```python
from build123d import *

# Parameters (mm, degrees)
SKETCH2_W           = 304.8
SKETCH2_H           = 304.8
BOSS_EXTRUDE1_DEPTH = 5.588
SKETCH4_W           = 1.27
SKETCH4_H           = 12.7
SKETCH4_W_2         = 12.7
SKETCH4_H_2         = 1.27
CUT_EXTRUDE1_DEPTH  = 432.088512656
SKETCH5_W           = 228.854
SKETCH5_H           = 12.954
CUT_EXTRUDE2_DEPTH  = 0.254
SKETCH6_R           = 16.002
SKETCH6_R_2         = 1.7
SKETCH6_R_3         = 1.96
CUT_EXTRUDE3_DEPTH  = 432.088512656
CUT_EXTRUDE4_DEPTH  = 432.088512656
SKETCH8_R           = 1.016
CUT_EXTRUDE5_DEPTH  = 432.088512656
SKETCH9_R           = 1.016
CUT_EXTRUDE6_DEPTH  = 432.088512656
BOSS_EXTRUDE3_REACH = 433.089
SKETCH10_W          = 236.011664121
SKETCH10_H          = 22.945578457


with BuildPart() as part:
    # Sketch2 → Boss-Extrude1 (new body)
    with BuildSketch(Plane(origin=(0, 0, 0), x_dir=(1, 0, 0), z_dir=(0, 1, 0))):
        with Locations((152.4, 152.4)):
            Rectangle(SKETCH2_W, SKETCH2_H)
    extrude(amount=BOSS_EXTRUDE1_DEPTH)

    # Sketch4 → Cut-Extrude1 (cut, through all)
    with BuildSketch(Plane(origin=(0, 5.588, 0), x_dir=(1, 0, 0), z_dir=(0, 1, 0))):
        with Locations((3.175, 8.89)):
            Rectangle(SKETCH4_W, SKETCH4_H)
        with Locations((295.91, 3.175)):
            Rectangle(SKETCH4_W_2, SKETCH4_H_2)
        with Locations((295.91, 6.985)):
            Rectangle(SKETCH4_W_2, SKETCH4_H_2)
    extrude(amount=-CUT_EXTRUDE1_DEPTH, mode=Mode.SUBTRACT)

    # Sketch5 → Cut-Extrude2 (cut)
    with BuildSketch(Plane(origin=(0, 5.588, 0), x_dir=(1, 0, 0), z_dir=(0, 1, 0))):
        with Locations((148.97354, 274.58924)):
            Rectangle(SKETCH5_W, SKETCH5_H)
    extrude(amount=-CUT_EXTRUDE2_DEPTH, mode=Mode.SUBTRACT)

    # Sketch6 → Cut-Extrude3 (cut, through all)
    with BuildSketch(Plane(origin=(0, 5.588, 0), x_dir=(1, 0, 0), z_dir=(0, 1, 0))):
        with Locations(Location((152.4799846, 126.1262654, 0), (0, 0, 270))):
            Circle(SKETCH6_R)
        with Locations(Location((31.75, 300.959132824, 0), (0, 0, 270))):
            Circle(SKETCH6_R_2)
        with Locations(Location((17.93875, 287.147882824, 0), (0, 0, 270))):
            Circle(SKETCH6_R_2)
        with Locations(Location((273.05, 300.959132824, 0), (0, 0, 270))):
            Circle(SKETCH6_R_2)
        with Locations(Location((286.86125, 287.147882824, 0), (0, 0, 270))):
            Circle(SKETCH6_R_2)
        with Locations(Location((286.86125, 222.906202824, 0), (0, 0, 270))):
            Circle(SKETCH6_R_2)
        with Locations(Location((273.05, 209.094952824, 0), (0, 0, 270))):
            Circle(SKETCH6_R_2)
        with Locations(Location((31.75, 209.094952824, 0), (0, 0, 270))):
            Circle(SKETCH6_R_2)
        with Locations(Location((17.93875, 222.906202824, 0), (0, 0, 270))):
            Circle(SKETCH6_R_2)
        with Locations(Location((38.1787654, 103.9330154, 0), (0, 0, 270))):
            Circle(SKETCH6_R_2)
        with Locations(Location((53.1330154, 88.9787654, 0), (0, 0, 270))):
            Circle(SKETCH6_R_2)
        with Locations(Location((251.6669846, 88.9787654, 0), (0, 0, 270))):
            Circle(SKETCH6_R_2)
        with Locations(Location((266.6212346, 103.9330154, 0), (0, 0, 270))):
            Circle(SKETCH6_R_2)
        with Locations(Location((266.6212346, 251.6669846, 0), (0, 0, 270))):
            Circle(SKETCH6_R_2)
        with Locations(Location((251.6669846, 236.7127346, 0), (0, 0, 270))):
            Circle(SKETCH6_R_2)
        with Locations(Location((53.1330154, 236.7127346, 0), (0, 0, 270))):
            Circle(SKETCH6_R_2)
        with Locations(Location((38.1787654, 251.6669846, 0), (0, 0, 270))):
            Circle(SKETCH6_R_2)
        with Locations(Location((130.6518596, 111.328047494, 0), (0, 0, 270))):
            Circle(SKETCH6_R_3)
        with Locations(Location((174.3081096, 111.328047494, 0), (0, 0, 270))):
            Circle(SKETCH6_R_3)
        with Locations(Location((187.4049846, 50.821596477, 0), (0, 0, 270))):
            Circle(SKETCH6_R_3)
        with Locations(Location((117.5549846, 50.821596477, 0), (0, 0, 270))):
            Circle(SKETCH6_R_3)
    extrude(amount=-CUT_EXTRUDE3_DEPTH, mode=Mode.SUBTRACT)

    # Sketch7 → Cut-Extrude4 (cut, through all)
    with BuildSketch(Plane(origin=(0, 5.588, 0), x_dir=(1, 0, 0), z_dir=(0, 1, 0))):
        with BuildLine():
            Line((145.076822752, 200.66), (132.376822752, 200.66))
            Line((132.376822752, 200.66), (132.376822752, 193.04))
            Line((132.376822752, 193.04), (145.076822752, 193.04))
            ThreePointArc((145.076822752, 193.04), (160.655, 196.85), (145.076822752, 200.66))
        make_face()
    extrude(amount=-CUT_EXTRUDE4_DEPTH, mode=Mode.SUBTRACT)

    # Sketch8 → Cut-Extrude5 (cut, through all)
    with BuildSketch(Plane(origin=(0, 5.588, 0), x_dir=(1, 0, 0), z_dir=(0, 1, 0))):
        with Locations(Location((206.6999846, 223.9950154, 0), (0, 0, 270))):
            Circle(SKETCH8_R)
        with Locations(Location((150.8199846, 223.9950154, 0), (0, 0, 270))):
            Circle(SKETCH8_R)
        with Locations(Location((94.9399846, 223.9950154, 0), (0, 0, 270))):
            Circle(SKETCH8_R)
    extrude(amount=-CUT_EXTRUDE5_DEPTH, mode=Mode.SUBTRACT)

    # Sketch9 → Cut-Extrude6 (cut, through all)
    with BuildSketch(Plane(origin=(0, 5.588, 0), x_dir=(1, 0, 0), z_dir=(0, 1, 0))):
        with Locations(Location((106.3, 242.18, 0), (0, 0, 270))):
            Circle(SKETCH9_R)
        with Locations(Location((106.3, 186.3, 0), (0, 0, 270))):
            Circle(SKETCH9_R)
        with Locations(Location((106.3, 130.42, 0), (0, 0, 270))):
            Circle(SKETCH9_R)
        with Locations(Location((198.5, 130.42, 0), (0, 0, 270))):
            Circle(SKETCH9_R)
        with Locations(Location((198.5, 186.3, 0), (0, 0, 270))):
            Circle(SKETCH9_R)
        with Locations(Location((198.5, 242.18, 0), (0, 0, 270))):
            Circle(SKETCH9_R)
    extrude(amount=-CUT_EXTRUDE6_DEPTH, mode=Mode.SUBTRACT)

    # Sketch10 → Boss-Extrude3 (add, up to next)
    with BuildSketch(Plane(origin=(0, 5.588, 0), x_dir=(1, 0, 0), z_dir=(0, 1, 0)), mode=Mode.PRIVATE) as boss_extrude3_sk1:
        with Locations((148.069627159, 275.695978824)):
            Rectangle(SKETCH10_W, SKETCH10_H)
    boss_extrude3_tool1 = extrude(boss_extrude3_sk1.sketch, amount=-BOSS_EXTRUDE3_REACH, mode=Mode.PRIVATE) - part.part
    add(boss_extrude3_tool1.solids().sort_by_distance((148.069627, 5.588, -275.695979))[0])


solid = part.part
```
Can you work these out from the model? Positions are in its coordinate system, mm. Round coordinates to 2 decimals unless told otherwise and drop trailing zeros. Loops run counter-clockwise (first coordinate to the right, second up) from the corner with the lowest first, then second, coordinate; pieces in that order, holes last. Notation, with made-up numbers: M 77.5,9.5 L 106.5,9.5 A18 ccw 106.5,38.5 Z; hole C 52,-27.5 d8. An arc over 180 degrees is marked long. Answer in a Markdown table with one row per item.
1. Thinking about a two-plate mould opening in X: for faces 1 (the face through (163.295, 2.833, -137.92)), 2 (the face through (150, 0, -155)), which applies, pulls with the +X half, pulls with the -X half, needs draft (parallel to the pull), parting line crosses it, or undercut?
Established:
| item | result |
|---|---|
| face 1 | undercut |
| face 2 | needs draft |
2. If we section it at A-A, the plane z = -125: Please give me the cut outline in (x, y).
Established:
| item | result |
|---|---|
| outline | M 0,0 L 136.52,0 L 136.52,5.59 L 0,5.59 Z; M 168.44,0 L 304.8,0 L 304.8,5.59 L 168.44,5.59 Z |
3. Please list where these lines run through material, in increasing order: line 1 (X direction, y = 2.1, z = -252); line 2 (X direction, y = 0.3, z = -286.5); line 3 (Z direction, x = 130.5, y = 4.3). Write a range as from..to.
Established:
| item | result |
|---|---|
| line 1 | 0..36.51, 39.85..264.95, 268.29..304.8 |
| line 2 | 0..16.37, 19.51..285.29, 288.43..304.8 |
| line 3 | -304.8..-113.28, -109.37..0 |
4. I'm going to push a flat-ended pin straight in: pin 1 Ø5 at (x, z) = (128, -97.5) entering from -Y. Where does the tip first touch, or does it pass through?
Established:
| item | result |
|---|---|
| pin 1 | y = 0 |
